```python
from build123d import *

# Parameters (mm, degrees)
F0_W     = 101.6
F0_H     = 25.4
F1_DEPTH = 76.2
F3_DEPTH = 25.4
F5_DEPTH = 25.4


with BuildPart() as f1:
    # F0 (on Front) → F1 (new body)
    with BuildSketch(Plane.XZ):
        with Locations((4.17847, -23.908158)):
            Rectangle(F0_W, F0_H)
    extrude(amount=F1_DEPTH)

    # F2 (on face) → F3 (join)
    with BuildSketch(Plane(origin=(0, 0, -36.608158), x_dir=(1, 0, 0), z_dir=(0, 0, -1))):
        Polygon((29.57847, 0), (54.97847, 0), (54.97847, 38.1), align=None)
    extrude(amount=F3_DEPTH)

    # F4 (on face) → F5 (join)
    with BuildSketch(Plane(origin=(0, 0, -36.608158), x_dir=(1, 0, 0), z_dir=(0, 0, -1))):
        Polygon((-46.62153, 76.2), (-46.62153, 0), (-21.22153, 0), (16.87847, 76.2), align=None)
    extrude(amount=F5_DEPTH)


solid = f1.part
```
Design review of the part built by this model. Coordinates are the model's own, in mm. A direction names the side the tool comes from. Give positions to 0.01 mm unless a question says otherwise; leave off trailing zeros. Order: outer loops, then holes, each group sorted by start corner. A loop starts at its lowest first (then second) coordinate and runs counter-clockwise, first axis right, second up. Notation, with made-up numbers: (23.25, -2.5) -> (57.25, -2.5) arc R25 cw to (57.25, 22.5) -> close; hole circle Ø1 at (77, -26). An arc over 180 degrees is marked (long way). Write item = value, one per line. Start each with the question number.
(1) For pin 1 (4 mm diameter, centred on x = 34, z = -56.5, fed in from +Y); pin 2 (8 mm diameter, centred on x = 28, z = -53, fed in from -Y); pin 3 (12 mm diameter, centred on x = 35, y = -32, fed in from -Z); pin 4 (6 mm diameter, centred on x = -11, z = -49, fed in from +Y), all flat-tipped, find the tip position at first contact; note any pin that passes through.
(2) For faces 1 (the face through (-2.438, -37.567, -49.13)), 2 (the face through (42.46, -19.32, -49.13)), 3 (the face through (-6, -76.2, -36)), list the 3-axis set-ups (+Z, -Z, +X, -X, +Y, -Y) from which the entire face can be reached by the end or side of a thin tool; tool diameter is ignored.
(3) Mouldability with a two-part tool opening along X and no side actions: class faces 4 (the face through (-46.622, -39, -36)), 5 (the face through (-22, -47, -62.008)), 6 (the face through (25, -38, -36.608)) as +X half, -X half, draft (parallel to the pull), parting line (faces both ways), or undercut.
(4) We need section A-A on z = -58. Write out the cut boundary in (x, y).
(5) To check wall thickness, follow line 1 along X through (y, z) = (-13, -52); line 2 along Z through (x, y) = (22, -28.5); line 3 along X through (y, z) = (-5, -48). State the ranges of each line that lie inside material, in increasing order.
(6) We need section B-B on y = -36. Write out the cut boundary in (x, z).
(7) We need section C-C on x = 31. Write out the cut boundary in (y, z).
(8) We need section D-D on y = -15. Write out the cut boundary in (x, z), plus the area to 3 significant figures.
Numbers:
q1.pin_1 = 0
q1.pin_2 = -3.63
q1.pin_3 = -36.61
q1.pin_4 = -14.44
q2.face_1 = -Z, +Y
q2.face_2 = -Z, -Y
q2.face_3 = +Z, -Z, +X, -X, -Y
q3.face_4 = -X half
q3.face_5 = draft
q3.face_6 = undercut
q4.outline = (-46.62, -76.2) -> (16.88, -76.2) -> (-21.22, 0) -> (-46.62, 0) -> close; (29.58, 0) -> (54.98, -38.1) -> (54.98, 0) -> close
q5.line_1 = -46.62 to -14.72, 38.25 to 54.98
q5.line_2 = -36.61 to -11.21
q5.line_3 = -46.62 to -18.72, 32.91 to 54.98
q6.outline = (-46.62, -62.01) -> (-3.22, -62.01) -> (-3.22, -36.61) -> (53.58, -36.61) -> (53.58, -62.01) -> (54.98, -62.01) -> (54.98, -11.21) -> (-46.62, -11.21) -> close
q7.outline = (-76.2, -36.61) -> (-2.13, -36.61) -> (-2.13, -62.01) -> (0, -62.01) -> (0, -11.21) -> (-76.2, -11.21) -> close
q8.outline = (-46.62, -62.01) -> (-13.72, -62.01) -> (-13.72, -36.61) -> (39.58, -36.61) -> (39.58, -62.01) -> (54.98, -62.01) -> (54.98, -11.21) -> (-46.62, -11.21) -> close
q8.area = 3,810 mm^2
